The listing builds one solid part. Answer for the finished solid, in the listing's coordinates (mm). Round coordinates to 2 decimals unless told otherwise and drop trailing zeros. Write each loop counter-clockwise with the first axis right and the second up, starting at its lowest first coordinate (ties: lowest second). Pieces come first, ordered by that corner, then holes. Notation, with made-up numbers: (61.5, -29.5) - (100.5, -29.5) arc R14 ccw to (100.5, -4.5) - close; hole circle Ø7 at (2, 70.25). An arc over 180 degrees is marked (long way). Return JSON: item names as keys, results as strings. Group by question number.
(1) This flat-tipped pin is pushed along its axis until it touches: pin 1 (1.8 mm diameter, centred on x = 12.5, z = 43.5, fed in from +Y). Where does it stop, or does it pass through?
(2) Section B-B, the plane y = 8.25 is taken. Give the number of separate pieces and of enclosed holes in the cut face, then the cut area to 3 significant figures.
(3) Determine the mould class of faces 1 (the cylindrical face through (-17.35, 7.05, 44.93)), 2 (the flat face through (0, 10.5, 42)), 3 (the cylindrical face through (13.4, 7, 5.7)), 4 (the cylindrical face through (12.44, 7.05, 25.5)) for opening direction Z: +Z half, -Z half, draft (parallel to the pull), parting line (faces both ways), or undercut.
(4) Find the intervals of material crossed by line 1 along X through (y, z) = (8.25, 43.5); line 2 along Z through (x, y) = (6, 8); line 3 along Z through (x, y) = (2, 8.75), in increasing order. Write a range as [from, to].
(5) Section A-A, the plane z = 24 is taken. Write down the section's boundary in (x, y).
(6) Section C-C, the plane x = -8.5 is taken. Write down the section's boundary in (y, z).
(7) Section D-D, the plane y = 4.5 is taken. Write down the section's boundary in (x, z), then the cut area to 3 significant figures.
Autodesk Inventor part; units mm, degrees
ref_plane "YZ Plane" through (0, 0, 0) normal (1, 0, 0) x (0, 1, 0)
ref_plane "XZ Plane" through (0, 0, 0) normal (0, 1, 0) x (-1, 0, 0)
ref_plane "XY Plane" through (0, 0, 0) normal (0, 0, 1) x (1, 0, 0)
sketch "Sketch1" plane through (0, 0, 0) normal (0, 0, 1) x (1, 0, 0)
  line L0 (-17.4973, 3.5) -> (-17.4973, 10.5)
  line L1 (-17.4973, 10.5) -> (17.5027, 10.5)
  line L2 (17.5027, 10.5) -> (17.5027, 3.5)
  line L3 (-17.4973, 3.5) -> (17.5027, 3.5)
  dimension "d50" = 35
  dimension "d51" = 7
extrude "Extrusion1" add sketch "Sketch1" along normal blind 48
sketch "Sketch4" plane through (-17.4973, 3.5, 0) normal (0, -1, 0) x (1, 0, 0)
  line L0 (35, 0) -> (0, 0)
  line L1 (35, 0) -> (35, 48)
  line L2 (0, 48) -> (35, 48)
  line L3 (0, 0) -> (0, 48)
  point P0 (5, 4.5)
  point P1 (5, 24)
  point P2 (5, 43.5)
  point P3 (30, 4.5)
  point P4 (30, 24)
  point P5 (30, 43.5)
  dimension "d52" = 4.5
  dimension "d53" = 4.5
  dimension "d54" = 5
  dimension "d55" = 5
  dimension "d56" = 24
hole "Hole2" at (-12.4973, 3.5, 4.5) at (-12.4973, 3.5, 24) at (-12.4973, 3.5, 43.5) at (12.5027, 3.5, 4.5) at (12.5027, 3.5, 24) at (12.5027, 3.5, 43.5) direction (0, 1, 0) diameter 3 end through all
sketch "Sketch5" plane through (17.5027, 3.5, 0) normal (1, 0, 0) x (0, 0, -1)
  circle A0 centre (-14.25, 7.1) radius 3
  circle A1 centre (-33.75, 7.1) radius 3
  line L0 (0, 7) -> (0, 0)
  line L1 (0, 7) -> (-48, 7)
  line L2 (-48, 0) -> (-48, 7)
  line L3 (0, 0) -> (-48, 0)
  point P0 (0, -3.5)
  dimension "d64" = 6
  dimension "d65" = 6
  dimension "d66" = 0.1
  dimension "d67" = 0.1
  dimension "d68" = 14.25
  dimension "d69" = 14.25
extrude "Extrusion3" cut sketch "Sketch5" against normal up to next contours A0 L1 | L1 A0 | L1 A1 | A1 L1
chamfer "Chamfer1" distance 3 angle 45 4 edges at (-17.4973, 7, 0) (-17.4973, 7, 48) (17.5027, 7, 48) (17.5027, 7, 0)
fillet "Fillet2" radius 2 8 edges at (-17.4973, 7, 3) (-14.4973, 7, 0) (-17.4973, 7, 45) (-14.4973, 7, 48) (14.5027, 7, 48) (17.5027, 7, 45) (14.5027, 7, 0) (17.5027, 7, 3)
equation "\"d69\" = d68"
properties part number "3DP_PLA_X_end_top_linear_shaft_clamp" material "ABS Plastic"
Working result:
{
 "1": {"pin 1": "passes through"},
 "2": {"separate pieces": "3", "enclosed holes": "6", "area": "1,360 mm^2"},
 "3": {"face 1": "+Z half", "face 2": "draft", "face 3": "undercut", "face 4": "undercut"},
 "4": {"line 1": "x = [-17.5, -14], [-11, 11], [14, 17.5]", "line 2": "z = [0, 12.75], [15.75, 32.25], [35.25, 48]", "line 3": "z = [0, 11.89], [16.61, 31.39], [36.11, 48]"},
 "5": {"outline": "(-17.5, 3.5) - (-14, 3.5) - (-14, 10.5) - (-17.5, 10.5) - close; (-11, 3.5) - (11, 3.5) - (11, 10.5) - (-11, 10.5) - close; (14, 3.5) - (17.5, 3.5) - (17.5, 10.5) - (14, 10.5) - close"},
 "6": {"outline": "(3.5, 0) - (10.5, 0) - (10.5, 11.25) arc R3 cw to (10.5, 17.25) - (10.5, 30.75) arc R3 cw to (10.5, 36.75) - (10.5, 48) - (3.5, 48) - close"},
 "7": {"outline": "(-17.5, 3.83) arc R2 ccw to (-16.91, 2.41) - (-15.08, 0.59) arc R2 ccw to (-13.67, 0) - (13.67, 0) arc R2 ccw to (15.09, 0.59) - (16.92, 2.41) arc R2 ccw to (17.5, 3.83) - (17.5, 44.17) arc R2 ccw to (16.92, 45.59) - (15.09, 47.41) arc R2 ccw to (13.67, 48) - (-13.67, 48) arc R2 ccw to (-15.08, 47.41) - (-16.91, 45.59) arc R2 ccw to (-17.5, 44.17) - close; hole circle Ø3 at (-12.5, 4.5); hole circle Ø3 at (-12.5, 24); hole circle Ø3 at (-12.5, 43.5); hole circle Ø3 at (12.5, 4.5); hole circle Ø3 at (12.5, 24); hole circle Ø3 at (12.5, 43.5)", "area": "1,620 mm^2"}
}
